```python
from build123d import *

# Parameters (mm, degrees)
F0_W     = 208.4420993924
F0_H     = 81.4700946212
F1_DEPTH = 25.4
F2_R     = 11.1076712279
F2_R_2   = 10.5439005504
F3_DEPTH = 50.8
F7_R     = 5.08


# Not quite as in the source:
# - the program builds the solid bodies; features that only make, move or delete a surface that nothing else refers to are left out


with BuildPart() as f1:
    # F0 (on Front) → F1 (new body)
    with BuildSketch(Plane.XZ):
        with Locations((-3.9001591504, -4.76687029)):
            Rectangle(F0_W, F0_H)
    extrude(amount=F1_DEPTH)

    # F2 (on face) → F3 (join)
    with BuildSketch(Plane.XZ.offset(25.4)):
        with Locations((-88.1870388985, -4.7668707557)):
            Circle(F2_R)
        with Locations((85.1535871625, 0)):
            Circle(F2_R_2)
    extrude(amount=F3_DEPTH)

    # F7
    f7_edges = [f1.edges().sort_by_distance(p)[0] for p in [
        (100.320891, -12.7, -45.501918),
        (-108.121209, -12.7, -45.501918),
        (-108.121209, -12.7, 35.968177),
        (100.320891, -12.7, 35.968177),
    ]]
    fillet(f7_edges, radius=F7_R)


solid = f1.part
```
The listing builds one solid part. Answer for the finished solid, in the listing's coordinates (mm). A direction names the side the tool comes from. Round coordinates to 2 decimals unless told otherwise and drop trailing zeros. Loops run counter-clockwise (first coordinate to the right, second up) from the corner with the lowest first, then second, coordinate; pieces in that order, holes last.
Q1. Section C-C, the plane x = -44 is taken. Determine the outline of the cut face in (y, z).
Q2. Section D-D, the plane z = 21 is taken. Determine the outline of the cut face in (x, y).
Q3. For a pull along X with two mould halves and no side action, classify faces 3 (the face through (-106.673, -12.878, 34.441)), 4 (the face through (-5, -13, -45.502)), 5 (the face through (-99.284, -50.444, -4.278)) as released by +X, released by -X, zero draft, split by the parting line, or undercut.
Q4. Section B-B, the plane y = -69.5 is taken. Determine the outline of the cut face in (x, z), then the cut area to 3 significant figures.
Q5. Which of the six approach directions +Z, -Z, +X, -X, +Y, -Y give full straight-line access (tool end or side, diameter ignored) to faces 1 (the face through (94.893, -50.444, -4.038)), 2 (the face through (-88, -76.2, -5))?
Q6. Find the intervals of material crossed by line 1 (X direction, y = -40, z = 4); line 2 (Y direction, x = -11, z = -40.5); line 3 (Z direction, x = -90.5, y = -38.5), in increasing order.
Q7. Given pin 1 Ø6 at (y, z) = (-58, 5) entering from +X; pin 2 Ø4 at (x, z) = (38.5, -31) entering from -Y; pin 3 Ø10 at (y, z) = (-37, -10) entering from -X, each flat-ended and moving along its own axis, determine where each tip first touches the part or whether it passes through.
Q8. Section A-A, the plane z = 2 is taken. Determine the outline of the cut face in (x, y), then the cut area to 3 significant figures.
Completed:
1. outline: (-25.4, -45.5) - (0, -45.5) - (0, 35.97) - (-25.4, 35.97) - close
2. outline: (-108.12, -25.4) - (100.32, -25.4) - (100.32, 0) - (-108.12, 0) - close
3. face 3: released by -X
3. face 4: zero draft
3. face 5: undercut
4. outline: circle Ø22.22 at (-88.19, -4.77); circle Ø21.09 at (85.15, 0)
4. area: 737 mm2
5. face 1: -Y
5. face 2: +Z, -Z, +X, -X, -Y
6. line 1: x = -95.01 to -81.37, 75.4 to 94.91
6. line 2: y = -25.4 to 0
6. line 3: z = -15.63 to 6.1
7. pin 1: stops at x = 95.51
7. pin 2: stops at y = -25.4
7. pin 3: stops at x = -99.29
8. outline: (-108.12, -25.4) - (-97, -25.4) - (-97, -76.2) - (-79.38, -76.2) - (-79.38, -25.4) - (74.8, -25.4) - (74.8, -76.2) - (95.51, -76.2) - (95.51, -25.4) - (100.32, -25.4) - (100.32, 0) - (-108.12, 0) - close
8. area: 7,240 mm2
